Autodesk Inventor part; units mm, degrees
ref_plane "YZ Plane" through (0, 0, 0) normal (1, 0, 0) x (0, 1, 0)
ref_plane "XZ Plane" through (0, 0, 0) normal (0, 1, 0) x (-1, 0, 0)
ref_plane "XY Plane" through (0, 0, 0) normal (0, 0, 1) x (1, 0, 0)
sketch "スケッチ1" plane through (0, 0, 0) normal (0, 1, 0) x (-1, 0, 0)
  circle A0 centre (0, 0) radius 6
  line L0 (3.3166, 5) -> (-3.3166, 5)
  line L1 (-3.3166, 5) -> (-3.3166, -5)
  line L2 (-3.3166, -5) -> (3.3166, -5)
  line L3 (3.3166, -5) -> (3.3166, 5)
  dimension "d0" = 12
  dimension "d1" = 10
extrude "押し出し1" add sketch "スケッチ1" along normal blind 15 contours A0 L3 | L3 L2 L1 L0 | L1 A0
sketch "スケッチ2" plane through (0, 0, 0) normal (0, -1, 0) x (1, 0, 0)
  circle A0 centre (0, 0) radius 2.5
  dimension "d4" = 5
extrude "押し出し2" add sketch "スケッチ2" along normal blind 1
sketch "スケッチ3" plane through (0, 0, 0) normal (0, -1, 0) x (1, 0, 0)
  line L0 (4, -0.75) -> (-4, -0.75)
  line L1 (-4, -0.75) -> (-4, 0.75)
  line L2 (-4, 0.75) -> (4, 0.75)
  line L3 (4, 0.75) -> (4, -0.75)
  line L4 (3.75, -0.75) -> (-3.75, -0.75)
  line L5 (-3.75, -0.75) -> (-3.75, 0.75)
  line L6 (-3.75, 0.75) -> (3.75, 0.75)
  line L7 (3.75, 0.75) -> (3.75, -0.75)
  point P0 (0, 0)
  point P1 (4, 0)
  point P2 (0, -0.75)
  point P3 (0, 0.75)
  dimension "d7" = 8
  dimension "d8" = 1.5
  dimension "d9" = 7.5
extrude "押し出し3" add sketch "スケッチ3" along normal blind 2 contours L0 L7 L2 L3 | L0 L1 L2 L5
sketch "スケッチ4" plane through (0, 15, 0) normal (0, 1, 0) x (1, 0, 0)
  line L0 (-6, 5) -> (6, 5)
  line L1 (6, 5) -> (6, -5)
  line L2 (6, -5) -> (-6, -5)
  line L3 (-6, -5) -> (-6, 5)
  line L4 (3.3166, 5) -> (-3.3166, 5)
  arc A0 (3.3166, -5) -> (3.3166, 5) centre (0, 0) ccw
  arc A1 (-3.3166, 5) -> (-3.3166, -5) centre (0, 0) ccw
  line L5 (-3.3166, -5) -> (3.3166, -5)
extrude "押し出し4" add sketch "スケッチ4" along normal blind 9
sketch "スケッチ5" plane through (0, 24, 0) normal (0, 1, 0) x (1, 0, 0)
  circle A0 centre (0, 0) radius 2
  dimension "d14" = 4
extrude "押し出し5" add sketch "スケッチ5" along normal blind 100
sketch "スケッチ6" plane through (0, 15, 0) normal (0, -1, 0) x (1, 0, 0)
  arc A0 (6, 0) -> (3.3166, 5) centre (0, 0) ccw
  line L0 (6, 5) -> (6, 0)
  line L1 (3.3166, 5) -> (6, 5)
  arc A1 (3.3166, -5) -> (6, 0) centre (0, 0) ccw
  line L2 (6, -5) -> (3.3166, -5)
  line L3 (6, 0) -> (6, -5)
  arc A2 (-6, 0) -> (-3.3166, -5) centre (0, 0) ccw
  line L4 (-6, -5) -> (-6, 0)
  line L5 (-3.3166, -5) -> (-6, -5)
  arc A3 (-3.3166, 5) -> (-6, 0) centre (0, 0) ccw
  line L6 (-6, 5) -> (-3.3166, 5)
  line L7 (-6, 0) -> (-6, 5)
  circle A4 centre (0, 0) radius 2
  line L8 (-6, -5) -> (-6, 5)
  line L9 (-6, 5) -> (6, 5)
  line L10 (6, 5) -> (6, -5)
  line L11 (6, -5) -> (-6, -5)
  circle A5 centre (0, 0) radius 5.75
  line L12 (3.2404, -4.75) -> (-3.2404, -4.75)
  line L13 (-3.2404, -4.75) -> (-3.2404, 4.75)
  line L14 (-3.2404, 4.75) -> (3.2404, 4.75)
  line L15 (3.2404, 4.75) -> (3.2404, -4.75)
  point P0 (-3.3166, -5)
  point P1 (3.3166, -5)
  dimension "d17" = 11.5
  dimension "d18" = 9.5
extrude "押し出し6" cut sketch "スケッチ6" along normal blind 0.5 contours A1 L11 A5 L9 A0 | A0 L1 L0 | L3 L2 A1 | A5 L14 L9 | L11 A5 L12 | A5 L11 A2 A3 L9 | A3 L7 L6 | L5 L4 A2
sketch "スケッチ7" plane through (0, 124, 0) normal (0, 1, 0) x (1, 0, 0)
  circle A0 centre (0, 0) radius 2
  circle A1 centre (0, 0) radius 1.5
  dimension "d21" = 3
extrude "押し出し7" cut sketch "スケッチ7" against normal blind 3
properties part number "motor_M4_100" material "アルミニウム 6061"
Build history of the part. All positions in model axes, mm. A direction names the side the tool comes from. Round coordinates to 2 decimals unless told otherwise and drop trailing zeros. Loops run counter-clockwise (first coordinate to the right, second up) from the corner with the lowest first, then second, coordinate; pieces in that order, holes last.
Item 1: Which spindle directions (+Z, -Z, +X, -X, +Y, -Y) get a long thin tool onto all of the face, cutting with end or side? Do faces 1 (the face through (-5.75, 14.75, -0.08)), 2 (the face through (-0.54, -0.49, 2.44)), 3 (the face through (6, 7, 0)). Say none if no direction does.
Item 2: Saw through at B-B (y = 30). List the corners of the cut face in (x, z), then the cut area to 3 significant figures.
Item 3: Saw through at C-C (y = 9). List the corners of the cut face in (x, z).
Item 4: Saw through at A-A (x = 0). List the corners of the cut face in (y, z).
Item 5: Two-plate mould, pull along Y, no slides. Class faces 4 (the face through (-0.1, 24, -2.3)), 5 (the face through (-6, 7, 0)), 6 (the face through (5.75, 14.75, 0.08)): released by +Y, released by -Y, zero draft, split by the parting line, or undercut.
Item 6: Pin check, flat tips, straight feed: P1, Ø0.8, axis at y = -1, z = -0.5, coming from the +X side; P2, Ø1.5, axis at x = -3.5, z = 1.5, coming from the -Y side; P3, Ø5.5, axis at x = 0.5, z = 1, coming from the -Y side. Stop position of each tip, or through.
Item 7: Drill centre lines: line 1 along Y through (x, z) = (4.75, 3.5); line 2 along Y through (x, z) = (2.25, 2); line 3 along Z through (x, y) = (0, 39). Where is each one in solid material? Low to high.
Worked answers:
1. face 1: -X
1. face 2: -Y
1. face 3: +X, -Y
2. outline: circle Ø4 at (0, 0)
2. area: 12.6 mm2
3. outline: (-3.32, -5) - (3.32, -5) arc R6 ccw to (3.32, 5) - (-3.32, 5) arc R6 ccw to start
4. outline: (-1, -2.5) - (0, -2.5) - (0, -5) - (14.5, -5) - (14.5, -4.75) - (15, -4.75) - (15, -5) - (24, -5) - (24, -2) - (121, -2) - (121, -1.5) - (124, -1.5) - (124, 1.5) - (121, 1.5) - (121, 2) - (24, 2) - (24, 5) - (15, 5) - (15, 4.75) - (14.5, 4.75) - (14.5, 5) - (0, 5) - (0, 2.5) - (-1, 2.5) - close
5. face 4: released by +Y
5. face 5: zero draft
5. face 6: undercut
6. P1: stops at x = 4
6. P2: stops at y = 0
6. P3: stops at y = -1
7. line 1: y = 0 to 14.5, 15 to 24
7. line 2: y = 0 to 24
7. line 3: z = -2 to 2
